from build123d import *

# Parameters (mm, degrees)
BOSS_EXTRUDE1_DEPTH = 76.2
FILLET1_R           = 4.826
SKETCH2_R           = 12.7
SKETCH2_R_2         = 10
CUT_EXTRUDE1_DEPTH  = 9.652
SKETCH3_R           = 3.5
CUT_EXTRUDE2_DEPTH  = 9.652


with BuildPart() as part:
    # Sketch1 → Boss-Extrude1 (new body, symmetric)
    with BuildSketch(Plane.XY):
        Polygon((-79.248, 88.9), (-88.9, 88.9), (-88.9, 0), (88.9, 0), (88.9, 88.9), (79.248, 88.9), (79.248, 5.334), (-79.248, 5.334), align=None)
    extrude(amount=BOSS_EXTRUDE1_DEPTH, both=True)

    # Fillet1
    fillet1_edges = [part.edges().sort_by_distance(p)[0] for p in [
        (-79.248, 5.334, 0),
        (79.248, 5.334, 0),
        (79.248, 88.9, 0),
        (-79.248, 88.9, 0),
    ]]
    fillet(fillet1_edges, radius=FILLET1_R)

    # Sketch2 → Cut-Extrude1 (cut)
    with BuildSketch(Plane(origin=(88.9, 0, 0), x_dir=(0, 0, -1), z_dir=(1, 0, 0))):
        with Locations((52.5, 50.8)):
            Circle(SKETCH2_R)
        with Locations((-52.5, 50.8)):
            Circle(SKETCH2_R)
        with Locations((0, 50.8)):
            Circle(SKETCH2_R_2)
    extrude(amount=-CUT_EXTRUDE1_DEPTH, mode=Mode.SUBTRACT)

    # Sketch3 → Cut-Extrude2 (cut)
    with BuildSketch(Plane.ZY.offset(88.9)):
        with Locations((-25.4, 25.4)):
            Circle(SKETCH3_R)
        with Locations((25.4, 25.4)):
            Circle(SKETCH3_R)
        with Locations((0, 25.4)):
            Circle(SKETCH3_R)
    extrude(amount=-CUT_EXTRUDE2_DEPTH, mode=Mode.SUBTRACT)


solid = part.part
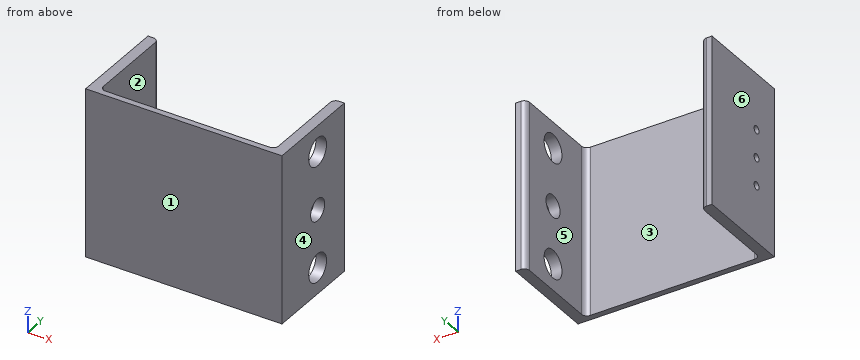
Geometry: final body of the model. Coordinates: model frame, mm. Face numbers are marked on the shaded views. A direction names the side the tool comes from. Coordinates: 2 decimals unless noted, no trailing zeros. Loops run counter-clockwise (first coordinate to the right, second up) from the corner with the lowest first, then second, coordinate; pieces in that order, holes last. Notation, with made-up numbers: (71.25, 79) - (109.25, 79) arc R37 cw to (109.25, 118) - close; hole circle Ø2 at (42, 54). An arc over 180 degrees is marked (long way). Put each result on its own line as item: value. Start each with the question number.
Q1. Pull-direction query (X, two-part tool) for the marked faces 1, 2, 3 and 4; classes: released by +X, released by -X, zero draft, split by the parting line, or undercut.
Q2. Cut plane B-B, the plane y = 25.4. Return loops of the section in (x, z), and give its area (3 significant figures).
Q3. Cut plane C-C, the plane y = 13.5. Return loops of the section in (x, z).
Q4. Line query: line 1 (Z direction, x = 82, y = 50); line 2 (Z direction, x = -86, y = 25); line 3 (X direction, y = 77, z = -36.5). Output: solid intervals per line, ascending.
Q5. Cut plane D-D, the plane z = 0. Return loops of the section in (x, y).
Q6. Cut plane A-A, the plane z = 25.4. Return loops of the section in (x, y), and give its area (3 significant figures).
Q7. Set-up query: the marked faces 5 and 6. Return all of +Z, -Z, +X, -X, +Y, -Y with unobstructed straight access to the full face (end or side cutting, diameter ignored); none if empty.
Q8. Pin query (flat end, axial travel): pin 1 Ø5.5 at (y, z) = (25.4, 0) entering from -X; pin 2 Ø1 at (x, z) = (57, 11.5) entering from -Y; pin 3 Ø15 at (y, z) = (50.8, 52.5) entering from +X; pin 4 Ø5 at (x, z) = (-3, -8) entering from +Y. Return the tip coordinate at first contact, or that it passes through.
Filled sheet:
1. face 1: zero draft
1. face 2: undercut
1. face 3: undercut
1. face 4: released by +X
2. outline: (-88.9, -76.2) - (-79.25, -76.2) - (-79.25, -28.9) - (-88.9, -28.9) - close; (-88.9, -21.9) - (-79.25, -21.9) - (-79.25, -3.5) - (-88.9, -3.5) - close; (-88.9, 3.5) - (-79.25, 3.5) - (-79.25, 21.9) - (-88.9, 21.9) - close; (-88.9, 28.9) - (-79.25, 28.9) - (-79.25, 76.2) - (-88.9, 76.2) - close; (79.25, -76.2) - (88.9, -76.2) - (88.9, 76.2) - (79.25, 76.2) - close
2. area: 2,740 mm²
3. outline: (-88.9, -76.2) - (-79.25, -76.2) - (-79.25, 76.2) - (-88.9, 76.2) - close; (79.25, -76.2) - (88.9, -76.2) - (88.9, 76.2) - (79.25, 76.2) - close
4. line 1: -76.2 to -65.17, -39.83 to -9.97, 9.97 to 39.83, 65.17 to 76.2
4. line 2: -76.2 to -28.88, -21.92 to -3.48, 3.48 to 21.92, 28.88 to 76.2
4. line 3: -88.9 to -79.25, 79.25 to 88.9
5. outline: (-88.9, 0) - (88.9, 0) - (88.9, 40.8) - (79.25, 40.8) - (79.25, 10.16) arc R4.83 cw to (74.42, 5.33) - (-74.42, 5.33) arc R4.83 cw to (-79.25, 10.16) - (-79.25, 21.9) - (-88.9, 21.9) - close; (-88.9, 28.9) - (-79.25, 28.9) - (-79.25, 84.07) arc R4.83 ccw to (-84.07, 88.9) - (-88.9, 88.9) - close; (79.25, 60.8) - (88.9, 60.8) - (88.9, 88.9) - (84.07, 88.9) arc R4.83 ccw to (79.25, 84.07) - close
6. outline: (-88.9, 0) - (88.9, 0) - (88.9, 88.9) - (84.07, 88.9) arc R4.83 ccw to (79.25, 84.07) - (79.25, 10.16) arc R4.83 cw to (74.42, 5.33) - (-74.42, 5.33) arc R4.83 cw to (-79.25, 10.16) - (-79.25, 21.9) - (-88.9, 21.9) - close; (-88.9, 28.9) - (-79.25, 28.9) - (-79.25, 84.07) arc R4.83 ccw to (-84.07, 88.9) - (-88.9, 88.9) - close
6. area: 2,490 mm²
7. face 5: +Z, -Z, +Y
7. face 6: +Z, -Z, -X, +Y, -Y
8. pin 1: x = 79.25
8. pin 2: y = 0
8. pin 3: x = -79.25
8. pin 4: y = 5.33
